Verification items for the finished model (mm, model axes). A direction names the side the tool comes from. Coordinates: 2 decimals unless noted, no trailing zeros. Write each loop counter-clockwise with the first axis right and the second up, starting at its lowest first coordinate (ties: lowest second). Pieces come first, ordered by that corner, then holes. Notation, with made-up numbers: (73.5, 72) -> (109.5, 72) arc R14 ccw to (109.5, 83) -> close; hole circle Ø4 at (31, 72.5). An arc over 180 degrees is marked (long way). Write item = value, one per line. Start each with the question number.
(1) Section check D-D (y = 31.5). Record the cut outline in (x, z).
(2) Gauge pin test, flat ends, axial feed: pin 1 Ø8 at (x, y) = (12, 14) entering from -Z; pin 2 Ø13.5 at (x, y) = (27.5, 16.5) entering from -Z; pin 3 Ø3 at (x, z) = (58, 5.5) entering from -Y; pin 4 Ø2 at (x, z) = (40.5, 4) entering from -Y. Record the tip position at first contact, or that the pin passes through.
(3) Section check A-A (y = 17.5). Record the cut outline in (x, z), plus the area to 4 significant figures.
(4) Section check C-C (y = 27.5). Record the cut outline in (x, z), plus the area to 3 significant figures.
(5) Set-up check for faces 5 (the face through (15, 32.5, 3)), 6 (the face through (4.973, 11.359, 1.726)), 7 (the face through (57, 13.75, 5)): record each of +Z, -Z, +X, -X, +Y, -Y from which the full face is reachable in a straight line by a thin tool's end or side.
(6) Mould release check, pull along X, two halves, no side actions. Record for faces 1 (the face through (23.886, 32.612, 3.549)), 2 (the face through (57, 21.25, 5)), 3 (the face through (40.114, 32.612, 3.549)), 4 (the face through (25, 6, 0)): released by +X, released by -X, zero draft, split by the parting line, or undercut.
(7) Section check B-B (x = 33). Record the cut outline in (y, z).
(8) Material ranges on probe 1 along Y at (x, z) = (56, 2.5); probe 2 along X at (y, z) = (28.5, 4.5); probe 3 along X at (y, z) = (18, 1), recorded low to high. Write a range as [from, to].
```python
from build123d import *
from build123d.topology import SkipClean

# Parameters (mm, degrees)
SKETCH1_R           = 2.75
BOSS_EXTRUDE1_DEPTH = 7
SKETCH2_R           = 12.1
CUT_EXTRUDE1_DEPTH  = 5.1
CUT_EXTRUDE2_DEPTH  = 3.5
FILLET1_R           = 5


with BuildPart() as part:
    # Sketch1 → Boss-Extrude1 (new body)
    with BuildSketch(Plane.XY):
        with BuildLine():
            Line((24.00000152, 32.500000075), (7.00000152, 32.500000075))
            ThreePointArc((7.00000152, 32.500000075), (2.050254052, 30.449747543), (1.52e-06, 25.500000075))
            Line((1.52e-06, 25.500000075), (1.52e-06, 9.500000075))
            ThreePointArc((1.52e-06, 9.500000075), (1.956143738, 4.646187277), (6.731286856, 2.50515966))
            Line((6.731286856, 2.50515966), (24.20077069, 1.834049785))
            ThreePointArc((24.20077069, 1.834049785), (27.99401413, 0.464681908), (32.00000152, 7.5e-08))
            Line((32.00000152, 7.5e-08), (32.00000152, 5.900000075))
            ThreePointArc((32.00000152, 5.900000075), (20.40000152, 17.500000075), (32.00000152, 29.100000075))
            Line((32.00000152, 29.100000075), (32.00000152, 34.500000075))
            ThreePointArc((32.00000152, 34.500000075), (27.876895894, 33.992422577), (24.00000152, 32.500000075))
        make_face()
        with Locations((7.00000152, 25.500000075)):
            Circle(SKETCH1_R, mode=Mode.SUBTRACT)
        with Locations((7.00000152, 9.500000075)):
            Circle(SKETCH1_R, mode=Mode.SUBTRACT)
    extrude(amount=BOSS_EXTRUDE1_DEPTH)

    # Sketch2 → Cut-Extrude1 (cut)
    with BuildSketch(Plane(origin=(0, 0, 0), x_dir=(-1, 0, 0), z_dir=(0, 0, -1))):
        with Locations((-32.00000152, 17.500000075)):
            Circle(SKETCH2_R)
    extrude(amount=-CUT_EXTRUDE1_DEPTH, mode=Mode.SUBTRACT)

    # Sketch3 → Cut-Extrude2 (cut)
    with BuildSketch(Plane.XY.offset(7)):
        Polygon((4.546262876, 29.750000075), (2.092524232, 25.500000075), (4.546262876, 21.250000075), (9.453740164, 21.250000075), (11.907478808, 25.500000075), (9.453740164, 29.750000075), align=None)
        Polygon((4.546262876, 13.750000075), (2.092524232, 9.500000075), (4.546262876, 5.250000075), (9.453740164, 5.250000075), (11.907478808, 9.500000075), (9.453740164, 13.750000075), align=None)
    extrude(amount=-CUT_EXTRUDE2_DEPTH, mode=Mode.SUBTRACT)

    # Fillet1
    fillet1_edges = [part.edges().sort_by_distance(p)[0] for p in [
        (24.00000152, 32.500000075, 3.5),
        (24.20077069, 1.834049785, 3.5),
    ]]
    fillet(fillet1_edges, radius=FILLET1_R)

    # Mirror1: part across plane


with BuildPart() as part_1:
    with SkipClean():  # the faces are left unmerged after this step: merging them gives an invalid solid
        add(part.part)
        add(part.part.mirror(Plane(origin=(32.00000152, 34.500000075, 7), x_dir=(0, 0, 1), z_dir=(-1, 0, 0))))


solid = part_1.part
```
Response:
q1.outline = (3.39, 0) -> (60.61, 0) -> (60.61, 7) -> (3.39, 7) -> close
q2.pin_1 = 0
q2.pin_2 = through
q2.pin_3 = 2.48
q2.pin_4 = 1.65
q3.outline = (0, 0) -> (19.9, 0) -> (19.9, 5.1) -> (20.4, 5.1) -> (20.4, 7) -> (0, 7) -> close; (43.6, 5.1) -> (44.1, 5.1) -> (44.1, 0) -> (64, 0) -> (64, 7) -> (43.6, 7) -> close
q3.area = 280.5 mm2
q4.outline = (0.29, 0) -> (5.11, 0) -> (5.11, 3.5) -> (3.25, 3.5) -> (3.25, 7) -> (0.29, 7) -> close; (8.89, 0) -> (25.19, 0) -> (25.19, 5.1) -> (26.12, 5.1) -> (26.12, 7) -> (10.75, 7) -> (10.75, 3.5) -> (8.89, 3.5) -> close; (37.88, 5.1) -> (38.81, 5.1) -> (38.81, 0) -> (55.11, 0) -> (55.11, 3.5) -> (53.25, 3.5) -> (53.25, 7) -> (37.88, 7) -> close; (58.89, 0) -> (63.71, 0) -> (63.71, 7) -> (60.75, 7) -> (60.75, 3.5) -> (58.89, 3.5) -> close
q4.area = 273 mm2
q5.face_5 = +Z, -Z, -X, +Y
q5.face_6 = +Z, -Z
q5.face_7 = +Z
q6.face_1 = released by -X
q6.face_2 = undercut
q6.face_3 = released by +X
q6.face_4 = zero draft
q7.outline = (0.03, 0) -> (5.44, 0) -> (5.44, 5.1) -> (5.94, 5.1) -> (5.94, 7) -> (0.03, 7) -> close; (29.06, 5.1) -> (29.56, 5.1) -> (29.56, 0) -> (34.47, 0) -> (34.47, 7) -> (29.06, 7) -> close
q8.probe_1 = [2.46, 6.94], [12.06, 22.94], [28.06, 32.5]
q8.probe_2 = [0.68, 3.82], [10.18, 26.96], [37.04, 53.82], [60.18, 63.32]
q8.probe_3 = [0, 19.91], [44.09, 64]
